Part model, mm, in its own coordinate system. Face numbers are marked on the shaded views. A direction names the side the tool comes from. Coordinates: 2 decimals unless noted, no trailing zeros. Write each loop counter-clockwise with the first axis right and the second up, starting at its lowest first coordinate (ties: lowest second). Pieces come first, ordered by that corner, then holes. Notation, with made-up numbers: (7, 32.25) -> (53, 32.25) arc R20 cw to (53, 63.25) -> close; hole circle Ø5 at (7, 9.5). An arc over 180 degrees is marked (long way). Write item = value, one per line. Start each with the question number.
Q1. Band-saw the part on D-D, the plane x = -39. List the corners of the cut face in (y, z).
Q2. Probe line 1 (Y direction, x = -38.75, z = 14); line 2 (X direction, y = 1.25, z = 11.5); line 3 (Z direction, x = -49, y = 0.5). List the from-to ranges inside material, lowest first.
Q3. Tool access for the marked faces 5 and 6: list every direction of +Z, -Z, +X, -X, +Y, -Y with a clear straight run to the whole face (end or side of a thin tool).
Q4. Pull direction X, two halves, no side cores. Call the marked faces 1, 2, 3 and 4: released by +X, released by -X, zero draft, split by the parting line, or undercut.
Q5. Band-saw the part on A-A, the plane x = -34. List the corners of the cut face in (y, z), plus the area to 3 significant figures.
Q6. Pin check, flat tips, straight feed: P1, Ø5, axis at x = -39.8, y = 4.03, coming from the +Z side; P2, Ø1.5, axis at x = -38.5, y = -2, coming from the -Z side; P3, Ø6, axis at x = -35, y = 9, coming from the -Z side. Stop position of each tip, or through.
Q7. Band-saw the part on B-B, the plane z = 9.75. List the corners of the cut face in (x, y).
Q8. Band-saw the part on C-C, the plane y = 2. List the corners of the cut face in (x, z), plus the area to 3 significant figures.
from build123d import *

# Parameters (mm, degrees)
CROQUIS1_W              = 20.5
CROQUIS1_H              = 17
CROQUIS1_W_2            = 18.5
CROQUIS1_H_2            = 15
SALIENTE_EXTRUIR1_DEPTH = 20
CROQUIS2_W              = 20.5
CROQUIS2_H              = 17
CROQUIS2_R              = 3.2
SALIENTE_EXTRUIR2_DEPTH = 1


with BuildPart() as part:
    # Croquis1 → Saliente-Extruir1 (new body)
    with BuildSketch(Plane.XY):
        with Locations((-39.801220416, 4.034561614)):
            Rectangle(CROQUIS1_W, CROQUIS1_H)
        with Locations((-39.801220416, 4.034561614)):
            Rectangle(CROQUIS1_W_2, CROQUIS1_H_2, mode=Mode.SUBTRACT)
    extrude(amount=SALIENTE_EXTRUIR1_DEPTH)

    # Croquis2 → Saliente-Extruir2 (add)
    with BuildSketch(Plane.XY.offset(20)):
        with Locations((-39.801220416, 4.034561614)):
            Rectangle(CROQUIS2_W, CROQUIS2_H)
        with Locations((-39.801220416, 4.034561614)):
            Circle(CROQUIS2_R, mode=Mode.SUBTRACT)
    extrude(amount=SALIENTE_EXTRUIR2_DEPTH)


solid = part.part
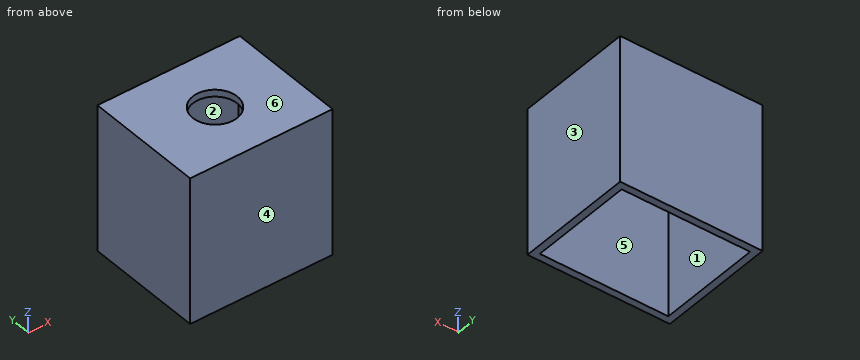
Ans:
q1.outline = (-4.47, 0) -> (-3.47, 0) -> (-3.47, 20) -> (0.94, 20) -> (0.94, 21) -> (-4.47, 21) -> close; (7.13, 20) -> (11.53, 20) -> (11.53, 0) -> (12.53, 0) -> (12.53, 21) -> (7.13, 21) -> close
q2.line_1 = -4.47 to -3.47, 11.53 to 12.53
q2.line_2 = -50.05 to -49.05, -30.55 to -29.55
q2.line_3 = 20 to 21
q3.face_5 = -Z
q3.face_6 = +Z, +X, -X, +Y, -Y
q4.face_1 = undercut
q4.face_2 = undercut
q4.face_3 = released by +X
q4.face_4 = zero draft
q5.outline = (-4.47, 0) -> (-3.47, 0) -> (-3.47, 20) -> (11.53, 20) -> (11.53, 0) -> (12.53, 0) -> (12.53, 21) -> (-4.47, 21) -> close
q5.area = 57.0 mm2
q6.P1 = through
q6.P2 = 20
q6.P3 = 0
q7.outline = (-50.05, -4.47) -> (-29.55, -4.47) -> (-29.55, 12.53) -> (-50.05, 12.53) -> close; hole (-49.05, -3.47) -> (-30.55, -3.47) -> (-30.55, 11.53) -> (-49.05, 11.53) -> close
q8.outline = (-50.05, 0) -> (-49.05, 0) -> (-49.05, 20) -> (-42.27, 20) -> (-42.27, 21) -> (-50.05, 21) -> close; (-37.33, 20) -> (-30.55, 20) -> (-30.55, 0) -> (-29.55, 0) -> (-29.55, 21) -> (-37.33, 21) -> close
q8.area = 55.6 mm2
